For this review, take the finished solid that the model builds, in its own axes (mm). Coordinates: 2 decimals unless noted, no trailing zeros. Write each loop counter-clockwise with the first axis right and the second up, starting at its lowest first coordinate (ties: lowest second). Pieces come first, ordered by that corner, then holes.
```python
from build123d import *

# Parameters (mm, degrees)
SKETCH1_R           = 11
SKETCH1_R_2         = 4
BOSS_EXTRUDE1_DEPTH = 7
FILLET1_R           = 1
FILLET2_R           = 1
FILLET3_R           = 0.5
FILLET4_R           = 0.5
SKETCH2_R           = 9
SKETCH2_R_2         = 6
CUT_EXTRUDE1_DEPTH  = 0.1
CUT_EXTRUDE2_START  = -0.1
SKETCH3_R           = 9.2
SKETCH3_R_2         = 6
CUT_EXTRUDE2_DEPTH  = 0.1


with BuildPart() as part:
    # Sketch1 → Boss-Extrude1 (new body)
    with BuildSketch(Plane.XY):
        with Locations(Location((0, 0, 0), (0, 0, 180))):
            Circle(SKETCH1_R)
        with Locations(Location((0, 0, 0), (0, 0, 180))):
            Circle(SKETCH1_R_2, mode=Mode.SUBTRACT)
    extrude(amount=BOSS_EXTRUDE1_DEPTH)

    # Fillet1
    fillet1_edges = [part.edges().sort_by_distance(p)[0] for p in [
        (11, 0, 7),
    ]]
    fillet(fillet1_edges, radius=FILLET1_R)

    # Fillet2
    fillet2_edges = [part.edges().sort_by_distance(p)[0] for p in [
        (11, 0, 0),
    ]]
    fillet(fillet2_edges, radius=FILLET2_R)

    # Fillet3
    fillet3_edges = [part.edges().sort_by_distance(p)[0] for p in [
        (4, 0, 7),
    ]]
    fillet(fillet3_edges, radius=FILLET3_R)

    # Fillet4
    fillet4_edges = [part.edges().sort_by_distance(p)[0] for p in [
        (4, 0, 0),
    ]]
    fillet(fillet4_edges, radius=FILLET4_R)

    # Sketch2 → Cut-Extrude1 (cut)
    with BuildSketch(Plane.XY.offset(7)):
        Circle(SKETCH2_R)
        Circle(SKETCH2_R_2, mode=Mode.SUBTRACT)
    extrude(amount=-CUT_EXTRUDE1_DEPTH, mode=Mode.SUBTRACT)

    # Sketch3 → Cut-Extrude2 (cut)
    with BuildSketch(Plane(origin=(0, 0, 0), x_dir=(-1, 0, 0), z_dir=(0, 0, -1)).offset(CUT_EXTRUDE2_START)):
        Circle(SKETCH3_R)
        with Locations(Location((0, 0, 0), (0, 0, 180))):
            Circle(SKETCH3_R_2, mode=Mode.SUBTRACT)
    extrude(amount=CUT_EXTRUDE2_DEPTH, mode=Mode.SUBTRACT)


solid = part.part
```
Q1. Add section C-C (z = 1.5). State the section outline as (x, y) points.
Ans:
outline: circle Ø22 at (0, 0); hole circle Ø8 at (0, 0)
Q2. Clearance check with flat-ended pins moving along their axes: pin 1 Ø5 at (x, y) = (0, 0) entering from +Z; pin 2 Ø1.5 at (y, z) = (-7.5, 4) entering from +X; pin 3 Ø6 at (x, y) = (-3, -3) entering from +Z; pin 4 Ø1.5 at (y, z) = (-8.5, 4) entering from -X. State where each tip first meets the part, or that it passes through.
Ans:
pin 1: passes through
pin 2: stops at x = 8.69
pin 3: stops at z = 7
pin 4: stops at x = -7.81
Q3. For probe 1 along Y at (x, z) = (0, 4); probe 2 along Z at (x, y) = (6.75, -3.5); probe 3 along Y at (x, z) = (0, 0.15), list the stretches that pass through material, from the lowest coordinate up.
Ans:
probe 1: y = -11 to -4, 4 to 11
probe 2: z = 0.1 to 6.9
probe 3: y = -10.53 to -4.14, 4.14 to 10.53
Q4. Draft analysis for pull direction X (two halves, no side actions). For faces 1 (the cylindrical face through (2.38, 10.74, 3.46)), 2 (the flat face through (2, -6, 6.9)), 3 (the flat face through (-2, -6, 0.1)), 4 (the flat face through (-3, 9, 0)), state which applies: +X half, -X half, draft (parallel to the pull), parting line (faces both ways), or undercut.
Ans:
face 1: parting line
face 2: undercut
face 3: undercut
face 4: draft
